Autodesk Inventor part; units mm, degrees
ref_plane "YZ Plane" through (0, 0, 0) normal (1, 0, 0) x (0, 1, 0)
ref_plane "XZ Plane" through (0, 0, 0) normal (0, 1, 0) x (-1, 0, 0)
ref_plane "XY Plane" through (0, 0, 0) normal (0, 0, 1) x (1, 0, 0)
sketch "Sketch1" plane through (0, 0, 0) normal (1, 0, 0) x (0, 1, 0)
  line L0 (5.7363, 8.6903) -> (-0.7637, 8.6903)
  line L1 (-0.7637, 8.6903) -> (-0.7637, 3.6903)
  line L2 (-0.7637, 3.6903) -> (2.5363, 3.6903)
  line L3 (2.5363, 3.6903) -> (2.5363, -3.3097)
  line L4 (2.5363, -3.3097) -> (-0.7637, -3.3097)
  line L5 (-0.7637, -3.3097) -> (-0.7637, -8.3097)
  line L6 (-0.7637, -8.3097) -> (5.7363, -8.3097)
  line L7 (5.7363, -8.3097) -> (5.7363, 8.6903)
  point P0 (0, 0)
  dimension "d0" = 17
  dimension "d1" = 3.3
  dimension "d2" = 6.5
  dimension "d3" = 5
  dimension "d4" = 7
extrude "Extrusion1" add sketch "Sketch1" along normal blind 22.5
sketch "Sketch2" plane through (0, 5.7363, 8.6903) normal (0, 1, 0) x (1, 0, 0)
  circle A0 centre (7.25, 2.5) radius 1
  circle A1 centre (15.25, 2.5) radius 1
  circle A2 centre (15.25, 14.5) radius 1
  circle A3 centre (7.25, 14.5) radius 1
  line L0 (0, 0) -> (22.5, 0)
  line L1 (22.5, 17) -> (22.5, 0)
  line L2 (0, 17) -> (0, 0)
  point P0 (0, 8.6903)
  dimension "d7" = 8
  dimension "d8" = 2
  dimension "d10" = 2
  dimension "d12" = 2
  dimension "d13" = 2
  dimension "d14" = 12
  dimension "d15" = 12
  dimension "d16" = 2.5
  dimension "d17" = 7.25
  dimension "d18" = 7.25
  dimension "d20" = 8
  dimension "d21" = 2.5
extrude "Extrusion2" cut sketch "Sketch2" against normal through all
properties part number "MGN7C_slider" material "ABS Plastic"
Verification items for the finished model (mm, model axes). A direction names the side the tool comes from. Coordinates: 2 decimals unless noted, no trailing zeros. Loops run counter-clockwise (first coordinate to the right, second up) from the corner with the lowest first, then second, coordinate; pieces in that order, holes last. Notation, with made-up numbers: (18, 89) -> (64, 89) arc R12 ccw to (64, 109) -> close; hole circle Ø2 at (-11, 69.25). An arc over 180 degrees is marked (long way). Answer as a JSON object with one key per item and string values. Group by question number.
Item 1: Sectioned sample at B-B on z = 6.5. Record the boundary of the cut face in (x, y).
Item 2: Sectioned sample at A-A on x = 7.25. Record the boundary of the cut face in (y, z).
Item 3: Scan lines: probe 1 along Z at (x, y) = (7.25, 2); probe 2 along X at (y, z) = (2, 6.25); probe 3 along Z at (x, y) = (7.25, 4.25). Record each from-to range of solid material in increasing order.
Item 4: Tool access check on faces 1 (the flat face through (11, 2.536, 0)), 2 (the cylindrical face through (16.174, 2.532, 6.573)). Record the directions out of +Z, -Z, +X, -X, +Y, -Y that give a thin tool (end or side, any length) a straight path to the whole face; none if there is none.
Item 5: Sectioned sample at C-C on x = 4. Record the boundary of the cut face in (y, z), plus the area to 3 significant figures.
Item 6: Mould release check, pull along X, two halves, no side actions. Record for faces 3 (the cylindrical face through (16.174, 2.532, -5.427)), 4 (the flat face through (11, -0.764, -6)), 5 (the flat face through (22.5, 3, 0)): +X half, -X half, draft (parallel to the pull), parting line (faces both ways), or undercut.
Item 7: Sectioned sample at D-D on y = 4. Record the boundary of the cut face in (x, z).
Evaluation:
{
 "1": {"outline": "(0, -0.76) -> (6.3, -0.76) -> (6.3, 5.74) -> (0, 5.74) -> close; (8.2, -0.76) -> (14.3, -0.76) -> (14.3, 5.74) -> (8.2, 5.74) -> close; (16.2, -0.76) -> (22.5, -0.76) -> (22.5, 5.74) -> (16.2, 5.74) -> close"},
 "2": {"outline": "(-0.76, -8.31) -> (5.74, -8.31) -> (5.74, -6.81) -> (-0.76, -6.81) -> close; (-0.76, -4.81) -> (5.74, -4.81) -> (5.74, 5.19) -> (-0.76, 5.19) -> (-0.76, 3.69) -> (2.54, 3.69) -> (2.54, -3.31) -> (-0.76, -3.31) -> close; (-0.76, 7.19) -> (5.74, 7.19) -> (5.74, 8.69) -> (-0.76, 8.69) -> close"},
 "3": {"probe 1": "z = -8.31 to -6.81, -4.81 to -3.31, 3.69 to 5.19, 7.19 to 8.69", "probe 2": "x = 0 to 6.25, 8.25 to 14.25, 16.25 to 22.5", "probe 3": "z = -8.31 to -6.81, -4.81 to 5.19, 7.19 to 8.69"},
 "4": {"face 1": "+X, -X, -Y", "face 2": "+Y, -Y"},
 "5": {"outline": "(-0.76, -8.31) -> (5.74, -8.31) -> (5.74, 8.69) -> (-0.76, 8.69) -> (-0.76, 3.69) -> (2.54, 3.69) -> (2.54, -3.31) -> (-0.76, -3.31) -> close", "area": "87.4 mm²"},
 "6": {"face 3": "undercut", "face 4": "draft", "face 5": "+X half"},
 "7": {"outline": "(0, -8.31) -> (22.5, -8.31) -> (22.5, 8.69) -> (0, 8.69) -> close; hole circle Ø2 at (7.25, -5.81); hole circle Ø2 at (7.25, 6.19); hole circle Ø2 at (15.25, -5.81); hole circle Ø2 at (15.25, 6.19)"}
}
